Geometry: final body of the model. Coordinates: model frame, mm. A direction names the side the tool comes from. Give positions to 0.01 mm unless a question says otherwise; leave off trailing zeros. Loops run counter-clockwise (first coordinate to the right, second up) from the corner with the lowest first, then second, coordinate; pieces in that order, holes last. Notation, with made-up numbers: (-7, -27.75) - (28, -27.75) arc R24 ccw to (28, 0.25) - close; hole circle Ø8 at (-25.75, -1.5). An arc over 180 degrees is marked (long way). Use one line per item in the form item = value.
```python
from build123d import *

# Parameters (mm, degrees)
BOSS_EXTRUDE1_DEPTH = 5.842
SKETCH2_R           = 7.6708
BOSS_EXTRUDE2_DEPTH = 14.224


with BuildPart() as part:
    # Sketch1 → Boss-Extrude1 (new body)
    with BuildSketch(Plane(origin=(0, 0, 0), x_dir=(1, 0, 0), z_dir=(0, 1, 0))):
        with BuildLine():
            Line((0, 10.95375), (57.9374, 10.95375))
            ThreePointArc((57.9374, 10.95375), (68.89115, 0), (57.9374, -10.95375))
            Line((57.9374, -10.95375), (0, -10.95375))
            ThreePointArc((0, -10.95375), (-10.95375, 0), (0, 10.95375))
        make_face()
    extrude(amount=BOSS_EXTRUDE1_DEPTH)

    # Sketch2 → Boss-Extrude2 (add)
    with BuildSketch(Plane(origin=(0, 5.842, 0), x_dir=(1, 0, 0), z_dir=(0, 1, 0))):
        with Locations((8.5979, 0)):
            Circle(SKETCH2_R)
        with Locations((49.3395, 0)):
            Circle(SKETCH2_R)
    extrude(amount=BOSS_EXTRUDE2_DEPTH)

    # Sketch3 → Revolve6 (revolve)
    with BuildSketch(Plane(origin=(0, 25.7048, 0), x_dir=(1, 0, 0), z_dir=(0, 1, 0))):
        with BuildLine():
            Line((-35.9537, -11.2776), (93.8911, -11.2776))
            ThreePointArc((93.8911, -11.2776), (101.865567436, -7.974467436), (105.1687, 0))
            Line((105.1687, 0), (-47.2313, 0))
            ThreePointArc((-47.2313, 0), (-43.928167436, -7.974467436), (-35.9537, -11.2776))
        make_face()
    revolve(axis=Axis((-35.9537, 25.7048, 0), (1, 0, 0)))


solid = part.part
```
(1) Pull-direction query (X, two-part tool) for faces 4 (the face through (41.676, 10.27, -0.337)), 5 (the face through (29, 3, 10.954)), 6 (the face through (-10.95, 2.88, 0.24)); classes: released by +X, released by -X, zero draft, split by the parting line, or undercut.
Solution:
face_4 = undercut
face_5 = zero draft
face_6 = released by -X
(2) Cut plane A-A (z = 0). Return the cut outline in (x, y), plus the area to 3 significant figures.
Solution:
outline = (-35.95, 14.43) - (0.93, 14.43) - (0.93, 5.84) - (-10.95, 5.84) - (-10.95, 0) - (68.89, 0) - (68.89, 5.84) - (57.01, 5.84) - (57.01, 14.43) - (93.89, 14.43) arc R11.28 ccw to (93.89, 36.98) - (-35.95, 36.98) arc R11.28 ccw to start; hole (16.27, 5.84) - (41.67, 5.84) - (41.67, 14.43) - (16.27, 14.43) - close
area = 4,060 mm2
(3) Material intervals for L1, parallel to Y at x = 26, z = -3.5; L2, parallel to X at y = 6.5, z = 2; L3, parallel to Z at x = 45.5, y = 5, sorted ascending. Write a range as from..to.
Solution:
L1 = 0..5.84, 14.98..36.43
L2 = 1.19..16, 41.93..56.74
L3 = -10.95..10.95
(4) Access query for faces 1 (the face through (29, 3, -10.954)), 2 (the face through (0.935, 10.27, -0.337)), 3 (the face through (68.89, 2.88, -0.24)). Directions: +Z, -Z, +X, -X, +Y, -Y. A direction counts if a zero-diameter tool reaches every point of the face in a straight line with its end or side. Return the directions, or none.
Solution:
face_1 = -Z, +X, -X, -Y
face_2 = none
face_3 = +X, -Y
(5) Pin query (flat end, axial travel): P1, Ø8, axis at x = 37, y = 23, coming from the -Z side; P2, Ø1, axis at x = 68.5, z = 8.5, coming from the +Y side; P3, Ø3, axis at x = 33.5, y = 3, coming from the -Z side; P4, Ø6.5, axis at x = 32, y = 3.5, coming from the +Z side. Return the tip coordinate at first contact, or that it passes through.
Solution:
P1 = -11.28
P2 = 33.65
P3 = -10.95
P4 = 10.95
(6) Cut plane D-D (x = 33). Return the cut outline in (y, z), plus the area to 3 significant figures.
Solution:
outline = (0, -10.95) - (5.84, -10.95) - (5.84, 10.95) - (0, 10.95) - close; circle Ø22.56 at (25.7, 0)
area = 528 mm2
(7) Cut plane B-B (y = 9.5). Return the cut outline in (x, z), plus the area to 3 significant figures.
Solution:
outline = circle Ø15.34 at (8.6, 0); circle Ø15.34 at (49.34, 0)
area = 370 mm2
(8) Cut plane C-C (z = 9). Return the cut outline in (x, y).
Solution:
outline = (-35.95, 18.91) - (93.89, 18.91) arc R6.8 ccw to (93.89, 32.5) - (-35.95, 32.5) arc R6.8 ccw to start; (-6.24, 0) - (64.18, 0) - (64.18, 5.84) - (-6.24, 5.84) - close
